Model file for the job. Use its own axes, mm. A direction names the side the tool comes from. Round coordinates to 2 decimals unless told otherwise and drop trailing zeros. Order: outer loops, then holes, each group sorted by start corner. A loop starts at its lowest first (then second) coordinate and runs counter-clockwise, first axis right, second up. Notation, with made-up numbers: (2.25, 11) - (15.25, 11) arc R23 cw to (15.25, 43) - close; hole circle Ø11 at (-6.75, 81). An arc over 180 degrees is marked (long way). Answer as CSV lines item,"result". Start each with the question number.
1. Wall check: line 1 along X through (y, z) = (-4.25, -23); line 2 along Z through (x, y) = (17.1, -8.75) (3 decimals); line 3 along Z through (x, y) = (-16.5, -5.6). Give the ranges that are in metal, low to high. Write a range as [from, to].
2. Band-saw the part on D-D on x = 4.5. List the corners of the cut face in (y, z), then the cut area to 3 significant figures.
3. Band-saw the part on C-C on z = -39.75. List the corners of the cut face in (x, y).
4. 3-axis set-ups, long thin cutter, end or side, ignore diameter. For faces 5 (the face through (16.99, -5.56, -43.15)), 6 (the face through (17.014, -11.237, -60.062)): which of +Z, -Z, +X, -X, +Y, -Y reach the whole face in a straight line?
5. Pull direction Y, two halves, no side cores. Call faces 1 (the face through (-16.986, -12.378, -73.557)), 2 (the face through (-16.99, -8.22, -36.09)), 3 (the face through (18, -4, -39)), 4 (the face through (17, -8.7, -38.8)): released by +Y, released by -Y, zero draft, split by the parting line, or undercut.
6. Band-saw the part on B-B on y = -8.75. List the corners of the cut face in (x, z) (3 decimals).
7. Band-saw the part on A-A on z = -66. List the corners of the cut face in (x, y).
8. Pin check, flat tips, straight feed: pin 1 Ø2 at (y, z) = (0, 0) entering from +X; pin 2 Ø1 at (x, z) = (17.5, -15.5) entering from -Y; pin 3 Ø1.1 at (y, z) = (-8.75, -39.75) entering from +X; pin 4 Ø6 at (x, y) = (-7, -8.5) entering from -Z. Stop position of each tip, or through.
```python
from build123d import *

# Parameters (mm, degrees)
SKETCH1_R                = 0.95
BOSS_EXTRUDE1_DEPTH      = 18
FILLET1_R                = 2
CUT_EXTRUDE1_DEPTH       = 83.531401045
CUT_EXTRUDE1_DEPTH_BACK  = 83.531401045
SKETCH2_W                = 32
SKETCH2_H                = 101.957647254
BOSS_EXTRUDE2_DEPTH      = 16
BOSS_EXTRUDE2_DEPTH_BACK = 18
SKETCH3_R                = 3.75


with BuildPart() as part:
    # Sketch1 → Boss-Extrude1 (new, symmetric)
    with BuildSketch(Plane(origin=(0, 0, 0), x_dir=(0, 0, -1), z_dir=(1, 0, 0))):
        with BuildLine():
            Line((0, 3.125), (31.1, 3.125))
            Line((31.1, 3.125), (46.5, 1.777674582))
            Line((46.5, 1.777674582), (63, -0.644122384))
            Line((63, -0.644122384), (70.830964262, -5.89639821))
            ThreePointArc((70.830964262, -5.89639821), (73.097482893, -6.816208289), (75.542765767, -6.754979641))
            Line((75.542765767, -6.754979641), (76.480663736, -6.535070013))
            ThreePointArc((76.480663736, -6.535070013), (79.183357394, -8.1108009), (77.757164464, -10.895303469))
            Line((77.757164464, -10.895303469), (69.23684377, -13.902469654))
            ThreePointArc((69.23684377, -13.902469654), (66.658598046, -14.216298138), (64.18928422, -13.41110961))
            Line((64.18928422, -13.41110961), (61.581493884, -11.871323024))
            ThreePointArc((61.581493884, -11.871323024), (60.039213852, -11.230596721), (58.380071029, -11.039801059))
            Line((58.380071029, -11.039801059), (37.117058695, -11.574311392))
            ThreePointArc((37.117058695, -11.574311392), (35.941440636, -11.021859195), (35.680027609, -9.749481703))
            Line((35.680027609, -9.749481703), (36.510915657, -6.64856529))
            ThreePointArc((36.510915657, -6.64856529), (36.260685553, -5.390573603), (35.110323209, -4.823277675))
            Line((35.110323209, -4.823277675), (7, -4.823277675))
            Line((7, -4.823277675), (-0.702972045, -3.044906452))
            ThreePointArc((-0.702972045, -3.044906452), (-3.104912049, 0.353760043), (0, 3.125))
        make_face()
        Circle(SKETCH1_R, mode=Mode.SUBTRACT)
        with Locations((77, -8.75)):
            Circle(SKETCH1_R, mode=Mode.SUBTRACT)
        with Locations((39.75, -8.75)):
            Circle(SKETCH1_R, mode=Mode.SUBTRACT)
        with Locations((44.1, -5.6)):
            Circle(SKETCH1_R, mode=Mode.SUBTRACT)
    extrude(amount=BOSS_EXTRUDE1_DEPTH, both=True)

    # Fillet1
    # the kernel refuses this fillet: 2 mm, written as the material it takes off along each edge
    with BuildSketch(Plane(origin=(18.569678042, -4.823277675, -7), x_dir=(0, 0, -1), z_dir=(-1, 0, 0))) as fillet1_piece_1:
        with BuildLine():
            CenterArc((FILLET1_R * 0.113935608302, -FILLET1_R), FILLET1_R, 90, 13)
            Line((-FILLET1_R * 0.111015446042, -FILLET1_R * 0.0256299352148), (0, 0))
            Line((0, 0), (FILLET1_R * 0.113935608302, 0))
        make_face()
    extrude(amount=37.139356083, mode=Mode.SUBTRACT)
    with BuildSketch(Plane(origin=(18.218304715, 3.125, -31.1), x_dir=(0, -0.08715574274766148, -0.9961946980917452), z_dir=(-1, 0, 0))) as fillet1_piece_2:
        with BuildLine():
            CenterArc((FILLET1_R * 0.0436609429085, FILLET1_R), FILLET1_R, 265, 5)
            Line((-FILLET1_R * 0.0434947998391, FILLET1_R * 0.00380530190825), (0, 0))
            Line((0, 0), (FILLET1_R * 0.0436609429085, 0))
        make_face()
    extrude(amount=36.436609429, mode=Mode.SUBTRACT)
    with BuildSketch(Plane(origin=(18.14621298, 1.777674582, -46.5), x_dir=(0, -0.1452196700772367, -0.9893994377513354), z_dir=(-1, 0, 0))) as fillet1_piece_3:
        with BuildLine():
            CenterArc((FILLET1_R * 0.0292425960983, FILLET1_R), FILLET1_R, 266.65, 3.35)
            Line((-FILLET1_R * 0.02919262642, FILLET1_R * 0.00170879761001), (0, 0))
            Line((0, 0), (FILLET1_R * 0.0292425960983, 0))
        make_face()
    extrude(amount=36.292425961, mode=Mode.SUBTRACT)
    with BuildSketch(Plane(origin=(19.131384491, -0.644122384, -63), x_dir=(0, -0.5570205743376945, -0.8304986934152907), z_dir=(-1, 0, 0))) as fillet1_piece_4:
        with BuildLine():
            CenterArc((FILLET1_R * 0.226276898255, FILLET1_R), FILLET1_R, 244.5, 25.5)
            Line((-FILLET1_R * 0.204234198553, FILLET1_R * 0.0974147156501), (0, 0))
            Line((0, 0), (FILLET1_R * 0.226276898255, 0))
        make_face()
    extrude(amount=38.262768983, mode=Mode.SUBTRACT)

    # Sketch2 → Cut-Extrude1 (cut, two sides: drawn at the far end of the back side and taken through both)
    with BuildSketch(Plane(origin=(0, 0, 0), x_dir=(1, 0, 0), z_dir=(0, 1, 0)).offset(-CUT_EXTRUDE1_DEPTH_BACK)):
        with Locations((0, 38.94963668)):
            Rectangle(SKETCH2_W, SKETCH2_H)
    extrude(amount=CUT_EXTRUDE1_DEPTH + CUT_EXTRUDE1_DEPTH_BACK, mode=Mode.SUBTRACT)


with BuildPart() as cut_extrude1_piece_1:
    # of the separate pieces the step leaves, piece 1, a body of its own (cut_extrude1_pieces)
    add(part.part.solids().sort_by_distance((-18, -4.823277675, -35.110323209))[0])



with BuildPart() as cut_extrude1_piece_2:
    # of the separate pieces the step leaves, piece 2, a body of its own (cut_extrude1_pieces)
    add(part.part.solids().sort_by_distance((16, -4.823277675, -35.110323209))[0])


with BuildPart() as cut_extrude1_piece_1_1:
    add(cut_extrude1_piece_1.part)

    add(cut_extrude1_piece_2.part)  # Boss-Extrude2 merges Cut-Extrude1 piece 2
    # Sketch3 → Boss-Extrude2 (add, two sides: drawn at the far end of the back side and taken through both)
    with BuildSketch(Plane(origin=(0, 0, 0), x_dir=(0, 0, -1), z_dir=(1, 0, 0)).offset(-BOSS_EXTRUDE2_DEPTH_BACK)):
        with Locations((58.65, -5.75)):
            Circle(SKETCH3_R)
    extrude(amount=BOSS_EXTRUDE2_DEPTH + BOSS_EXTRUDE2_DEPTH_BACK)


solid = cut_extrude1_piece_1_1.part
```
Reply:
1,line 1,"x = [-18, -16], [16, 18]"
1,line 2,"z = [-79.275, -77.95], [-76.05, -40.7], [-38.8, -35.948]"
1,line 3,"z = [-70.39, -45.05], [-43.15, -36.39]"
2,outline,"circle Ø7.5 at (-5.75, -58.65)"
2,area,"44.2 mm2"
3,outline,"(-18, -11.51) - (-16, -11.51) - (-16, -9.7) - (-18, -9.7) - close; (-18, -7.8) - (-16, -7.8) - (-16, 2.37) - (-18, 2.37) - close; (16, -11.51) - (18, -11.51) - (18, -9.7) - (16, -9.7) - close; (16, -7.8) - (18, -7.8) - (18, 2.37) - (16, 2.37) - close"
4,face 5,"+X, -X"
4,face 6,"+X, -X, -Y"
5,face 1,"released by -Y"
5,face 2,"undercut"
5,face 3,"zero draft"
5,face 4,"undercut"
6,outline,"(-18, -79.275) - (-16, -79.275) - (-16, -77.95) - (-18, -77.95) - close; (-18, -76.05) - (-16, -76.05) - (-16, -60.9) - (16, -60.9) - (16, -76.05) - (18, -76.05) - (18, -40.7) - (16, -40.7) - (16, -56.4) - (-16, -56.4) - (-16, -40.7) - (-18, -40.7) - close; (-18, -38.8) - (-16, -38.8) - (-16, -35.948) - (-18, -35.948) - close; (16, -79.275) - (18, -79.275) - (18, -77.95) - (16, -77.95) - close; (16, -38.8) - (18, -38.8) - (18, -35.948) - (16, -35.948) - close"
7,outline,"(-18, -14.12) - (-16, -14.12) - (-16, -2.66) - (-18, -2.66) - close; (16, -14.12) - (18, -14.12) - (18, -2.66) - (16, -2.66) - close"
8,pin 1,"stops at x = 18"
8,pin 2,"stops at y = -4.82"
8,pin 3,"passes through"
8,pin 4,"stops at z = -62.4"
